from build123d import *

# Parameters (mm, degrees)
F0_W     = 50.8
F0_H     = 25.4
F1_DEPTH = 12.7
F2_R     = 4.826
F3_DEPTH = 6.35


# Not quite as in the source:
# - a feature names something its author has since deleted; it is built from what else it names


with BuildPart() as f1:
    # F0 (on Top) → F1 (new body)
    with BuildSketch(Plane.XY):
        Rectangle(F0_W, F0_H)
        Polygon((37.9070584633, 10.4946681436), (25.4, 12.7), (25.4, -12.7), (37.9070584633, -14.9053318564), (37.9070584633, -2.2053318564), align=None)
    extrude(amount=-F1_DEPTH)

    # F2 (on face) → F3 (join)
    with BuildSketch(Plane.YZ.offset(37.9070584633)):
        with Locations((-2.2053318564, -6.35)):
            Circle(F2_R)
    extrude(amount=F3_DEPTH)


solid = f1.part
Read the model definition and answer for the solid it produces. Units are mm, in the model's axes. A direction names the side the tool comes from. Coordinates: 2 decimals unless noted, no trailing zeros. Order: outer loops, then holes, each group sorted by start corner. A loop starts at its lowest first (then second) coordinate and runs counter-clockwise, first axis right, second up. Notation, with made-up numbers: M 86,-26 L 127,-26 A12 cw 127,-9 Z; hole C -18.5,-32 d5. An arc over 180 degrees is marked long. Put each result on its own line as item: value. Start each with the question number.
Item 1: Section B-B, the plane y = -8.5 is taken. Determine the outline of the cut face in (x, z).
Item 2: Given pin 1 Ø4 at (x, z) = (-4.5, -5) entering from -Y; pin 2 Ø1 at (x, y) = (19.5, 3.5) entering from +Z, each flat-ended and moving along its own axis, determine where each tip first touches the part or whether it passes through.
Item 3: Section D-D, the plane z = -2.5 is taken. Determine the outline of the cut face in (x, y), plus the area to 3 significant figures.
Item 4: Section A-A, the plane z = -6.35 is taken. Determine the outline of the cut face in (x, y), plus the area to 3 significant figures.
Item 5: Consider probe 1 along X at (y, z) = (7.75, -7.5); probe 2 along Y at (x, z) = (1, -10); probe 3 along Y at (x, z) = (40.5, -6.25). Determine where each line is inside the solid, lowest interval first. Write a range as [from, to].
Item 6: Section C-C, the plane x = 9 is taken. Determine the outline of the cut face in (y, z).
Item 7: For faces 1 (the face through (0, -12.7, -6)), 2 (the face through (41.04, 0.39, -2.28)), 3 (the face through (6, -1, -12.7)), determine the directions among +Z, -Z, +X, -X, +Y, -Y from which every point of the face is accessible in a straight line to the end or side of a thin tool.
Computed:
1. outline: M -25.4,-12.7 L 37.91,-12.7 L 37.91,0 L -25.4,0 Z
2. pin 1: stops at y = -12.7
2. pin 2: stops at z = 0
3. outline: M -25.4,-12.7 L 25.4,-12.7 L 37.91,-14.91 L 37.91,-5.12 L 44.26,-5.12 L 44.26,0.7 L 37.91,0.7 L 37.91,10.49 L 25.4,12.7 L -25.4,12.7 Z
3. area: 1,640 mm2
4. outline: M -25.4,-12.7 L 25.4,-12.7 L 37.91,-14.91 L 37.91,-7.03 L 44.26,-7.03 L 44.26,2.62 L 37.91,2.62 L 37.91,10.49 L 25.4,12.7 L -25.4,12.7 Z
4. area: 1,670 mm2
5. probe 1: x = [-25.4, 37.91]
5. probe 2: y = [-12.7, 12.7]
5. probe 3: y = [-7.03, 2.62]
6. outline: M -12.7,-12.7 L 12.7,-12.7 L 12.7,0 L -12.7,0 Z
7. face 1: +Z, -Z, -X, -Y
7. face 2: +X
7. face 3: -Z, +X, -X, +Y, -Y
